Input: part model. Units: mm. Frame: model coordinates. Give positions to 0.01 mm unless a question says otherwise; leave off trailing zeros. Order: outer loops, then holes, each group sorted by start corner. A loop starts at its lowest first (then second) coordinate and runs counter-clockwise, first axis right, second up. Notation, with made-up numbers: (81.25, 78) - (130.25, 78) arc R7 cw to (130.25, 91) - close; hole circle Ø9 at (66.5, -22). An arc over 180 degrees is marked (long way). Answer in a Markdown table with one row per item. Add a question column.
1. Contact query for flat-ended pins moving along their axis: pin 1 (5 mm diameter, centred on x = 11.5, z = 370, fed in from -Y); pin 2 (6 mm diameter, centred on x = 9.5, y = -446, fed in from +Z); pin 3 (8 mm diameter, centred on x = 18.5, z = 645, fed in from +Y). Output: stop coordinate, or through.
2. Section query A-A on z = 191. Return loops of the section in (x, y).
3. Ray query, line 1 (Y direction, x = 14.5, z = 168); line 2 (Y direction, x = 4.25, z = 176.5); line 3 (Z direction, x = 18.25, y = -366.5). Return the intervals inside material, ascending. Write a range as [from, to].
4. Section query D-D on y = -386.5. Return loops of the section in (x, z), and give its area (3 significant figures).
5. Section query C-C on y = -519. Return loops of the section in (x, z).
6. Section query B-B on x = 18.5. Return loops of the section in (y, z), and give its area (3 significant figures).
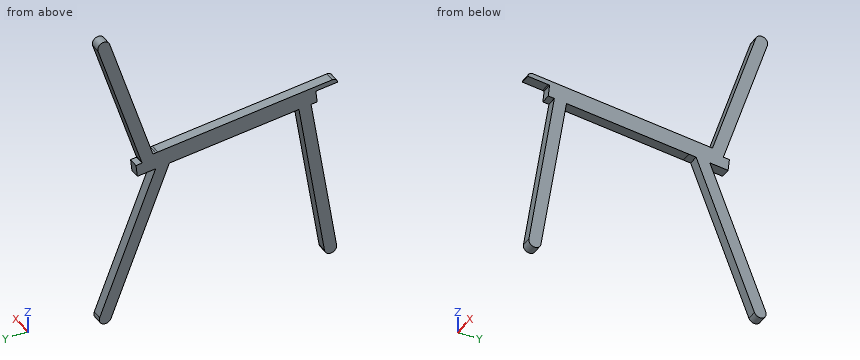
```python
from build123d import *

# Parameters (mm, degrees)
F1_DEPTH = 25


with BuildPart() as f1:
    # F0 (on Right) → F1 (new body)
    with BuildSketch(Plane.YZ):
        with BuildLine():
            Line((24.602603, 19.439522), (-112.858058, 370.132945))
            Line((-112.858058, 370.132945), (-113.312946, 370.183488))
            Line((-113.312946, 370.183488), (-117.698107, 370.670728))
            Line((-117.698107, 370.670728), (-146.547582, 373.876225))
            Line((-146.547582, 373.876225), (-3.328384, 8.491464))
            ThreePointArc((-3.328384, 8.491464), (16.111139, 0), (24.602603, 19.439522))
        make_face()
        with BuildLine():
            Line((-527.65253, 12.470365), (-464.846842, 409.24281))
            Line((-464.846842, 409.24281), (-494.695385, 412.559315))
            Line((-494.695385, 412.559315), (-557.283606, 17.160711))
            ThreePointArc((-557.283606, 17.160711), (-544.813241, 0), (-527.65253, 12.470365))
        make_face()
        with BuildLine():
            ThreePointArc((28.543336, 730.765391), (18.888972, 749.654363), (0, 740))
            Line((0, 740), (-106.229303, 411.654881))
            ThreePointArc((-106.229303, 411.654881), (-106.738574, 409.286215), (-107.713254, 407.068124))
            Line((-107.713254, 407.068124), (-110, 400))
            Line((-110, 400), (-79.563133, 396.618126))
            Line((-79.563133, 396.618126), (-78.468997, 400))
            Line((-78.468997, 400), (28.543336, 730.765391))
        make_face()
        Polygon((-164.400516, 375.859885), (-161.087571, 405.676397), (-506.290695, 444.032299), (-509.603641, 414.215787), (-494.695385, 412.559315), (-464.846842, 409.24281), align=None)
        with BuildLine():
            Line((-107.713254, 407.068124), (-106.229303, 411.654881))
            Line((-106.229303, 411.654881), (-113.12206, 412.420742))
            Line((-113.12206, 412.420742), (-118.155908, 412.980059))
            Line((-118.155908, 412.980059), (-546.748217, 460.601427))
            ThreePointArc((-546.748217, 460.601427), (-555.569736, 458.045247), (-560, 450))
            Line((-560, 450), (-510, 444.444444))
            Line((-510, 444.444444), (-506.290695, 444.032299))
            Line((-506.290695, 444.032299), (-161.087571, 405.676397))
            Line((-161.087571, 405.676397), (-121.926605, 401.325178))
            Line((-121.926605, 401.325178), (-119.481086, 401.053454))
            ThreePointArc((-119.481086, 401.053454), (-112.694575, 402.294843), (-107.713254, 407.068124))
        make_face()
        Polygon((-79.563133, 396.618126), (-110, 400), (-119.481086, 401.053454), (-121.926605, 401.325178), (-161.087571, 405.676397), (-164.400516, 375.859885), (-146.547582, 373.876225), (-117.698107, 370.670728), (-113.312946, 370.183488), (-112.858058, 370.132945), (-67.967822, 365.145141), (-64.654877, 394.961653), align=None)
        with BuildLine():
            ThreePointArc((-107.713254, 407.068124), (-106.738574, 409.286215), (-106.229303, 411.654881))
            Line((-106.229303, 411.654881), (-107.713254, 407.068124))
        make_face()
        with BuildLine():
            Line((-110, 400), (-107.713254, 407.068124))
            ThreePointArc((-107.713254, 407.068124), (-112.694575, 402.294843), (-119.481086, 401.053454))
            Line((-119.481086, 401.053454), (-110, 400))
        make_face()
    extrude(amount=F1_DEPTH)


solid = f1.part
```
Answer:
| question | item | result |
|---|---|---|
| 1 | pin 1 | stops at y = -501.83 |
| 1 | pin 2 | stops at z = 449.74 |
| 1 | pin 3 | stops at y = 2.09 |
| 2 | outline | (0, -529.77) - (25, -529.77) - (25, -499.39) - (0, -499.39) - close; (0, -74.87) - (25, -74.87) - (25, -42.64) - (0, -42.64) - close |
| 3 | line 1 | y = [-533.41, -503.03], [-65.85, -33.63] |
| 3 | line 2 | y = [-532.06, -501.69], [-69.18, -36.96] |
| 3 | line 3 | z = [398.32, 440.57] |
| 4 | outline | (0, 400.54) - (25, 400.54) - (25, 442.8) - (0, 442.8) - close |
| 4 | area | 1,060 mm² |
| 5 | outline | (0, 67.13) - (25, 67.13) - (25, 259.02) - (0, 259.02) - close; (0, 445.44) - (25, 445.44) - (25, 457.52) - (0, 457.52) - close |
| 6 | outline | (-560, 450) - (-506.29, 444.03) - (-509.6, 414.22) - (-494.7, 412.56) - (-557.28, 17.16) arc R15 ccw to (-527.65, 12.47) - (-464.85, 409.24) - (-146.55, 373.88) - (-3.33, 8.49) arc R15 ccw to (24.6, 19.44) - (-112.86, 370.13) - (-67.97, 365.15) - (-64.65, 394.96) - (-79.56, 396.62) - (28.54, 730.77) arc R15 ccw to (0, 740) - (-106.23, 411.65) - (-113.12, 412.42) - (-118.16, 412.98) - (-546.75, 460.6) arc R12 ccw to start |
| 6 | area | 54,000 mm² |
